Here's how the part is built. I have some questions about the finished solid (model axes, mm). Round coordinates to 2 decimals unless told otherwise and drop trailing zeros. Order: outer loops, then holes, each group sorted by start corner. A loop starts at its lowest first (then second) coordinate and runs counter-clockwise, first axis right, second up. Notation, with made-up numbers: (-23, -2) -> (6, -2) arc R18 cw to (6, 16) -> close; hole circle Ø1 at (-16, 71.25). An arc over 180 degrees is marked (long way). Use a Markdown table: item, result. Add a question column.
from build123d import *

# Parameters (mm, degrees)
SKETCH1_W           = 83
SKETCH1_H           = 327.5
BOSS_EXTRUDE1_DEPTH = 2
SKETCH2_R           = 1.6
CUT_EXTRUDE1_DEPTH  = 2
SKETCH3_R           = 1.93
CUT_EXTRUDE2_DEPTH  = 2
SKETCH4_W           = 116.407651787
SKETCH4_H           = 181.18090695
CUT_EXTRUDE3_DEPTH  = 10


with BuildPart() as part:
    # Sketch1 → Boss-Extrude1 (new body)
    with BuildSketch(Plane.XY):
        with Locations((41.5, 163.75)):
            Rectangle(SKETCH1_W, SKETCH1_H)
    extrude(amount=BOSS_EXTRUDE1_DEPTH)

    # Sketch2 → Cut-Extrude1 (cut)
    with BuildSketch(Plane.XY.offset(2)):
        with Locations((3.2, 314.9)):
            Circle(SKETCH2_R)
        with Locations((3.2, 308.5)):
            Circle(SKETCH2_R)
        with Locations((79.8, 314.9)):
            Circle(SKETCH2_R)
        with Locations((79.8, 308.5)):
            Circle(SKETCH2_R)
        with Locations((3.2, 240.925)):
            Circle(SKETCH2_R)
        with Locations((3.2, 234.525)):
            Circle(SKETCH2_R)
        with Locations((79.8, 240.925)):
            Circle(SKETCH2_R)
        with Locations((79.8, 234.525)):
            Circle(SKETCH2_R)
        with Locations((3.2, 166.95)):
            Circle(SKETCH2_R)
        with Locations((3.2, 160.55)):
            Circle(SKETCH2_R)
        with Locations((79.8, 166.95)):
            Circle(SKETCH2_R)
        with Locations((79.8, 160.55)):
            Circle(SKETCH2_R)
        with Locations((3.2, 92.975)):
            Circle(SKETCH2_R)
        with Locations((3.2, 86.575)):
            Circle(SKETCH2_R)
        with Locations((79.8, 92.975)):
            Circle(SKETCH2_R)
        with Locations((79.8, 86.575)):
            Circle(SKETCH2_R)
        with Locations((3.2, 19)):
            Circle(SKETCH2_R)
        with Locations((3.2, 12.6)):
            Circle(SKETCH2_R)
        with Locations((79.8, 19)):
            Circle(SKETCH2_R)
        with Locations((79.8, 12.6)):
            Circle(SKETCH2_R)
    extrude(amount=-CUT_EXTRUDE1_DEPTH, mode=Mode.SUBTRACT)

    # Sketch3 → Cut-Extrude2 (cut)
    with BuildSketch(Plane.XY.offset(2)):
        with Locations((41.5, 322.524)):
            Circle(SKETCH3_R)
        with Locations((41.5, 4.976)):
            Circle(SKETCH3_R)
    extrude(amount=-CUT_EXTRUDE2_DEPTH, mode=Mode.SUBTRACT)

    # Sketch4 → Cut-Extrude3 (cut)
    with BuildSketch(Plane.XY.offset(2)):
        with Locations((24.796174107, 254.340453475)):
            Rectangle(SKETCH4_W, SKETCH4_H)
    extrude(amount=-CUT_EXTRUDE3_DEPTH, mode=Mode.SUBTRACT)


solid = part.part
(1) If we mould it in two halves opening along Y, with no side actions, what happens to faces 1 (the flat face through (41, 83, 2)), 2 (the cylindrical face through (2.85, 11.04, 1.01))? For each: pulls with the +Y half, pulls with the -Y half, needs draft (parallel to the pull), parting line crosses it, or undercut.
(2) I want a section at B-B on y = 12.6. List the corners of the cut face in (x, z) for me.
(3) Please list where these lines run through material, in increasing order: probe 1 along Y at (x, z) = (3.2, 1.1) (3 decimals); probe 2 along X at (y, z) = (160.55, 1.35); probe 3 along Y at (x, z) = (78.5, 0.55). Write a range as from..to.
(4) I want a section at A-A on x = 79.8. List the corners of the cut face in (y, z) for me (3 decimals), and give its area (4 significant figures).
(5) I'm going to push a flat-ended pin straight in: P1, Ø2.5, axis at x = 3.2, y = 86.575, coming from the -Z side. Where does the tip first touch, or does it pass through?
Output:
| question | item | result |
|---|---|---|
| 1 | face 1 | needs draft |
| 1 | face 2 | undercut |
| 2 | outline | (0, 0) -> (1.6, 0) -> (1.6, 2) -> (0, 2) -> close; (4.8, 0) -> (78.2, 0) -> (78.2, 2) -> (4.8, 2) -> close; (81.4, 0) -> (83, 0) -> (83, 2) -> (81.4, 2) -> close |
| 3 | probe 1 | 0..11, 14.2..17.4, 20.6..84.975, 88.175..91.375, 94.575..158.95, 162.15..163.75 |
| 3 | probe 2 | 0..1.6, 4.8..78.2, 81.4..83 |
| 3 | probe 3 | 0..11.67, 13.53..18.07, 19.93..85.64, 87.51..92.04, 93.91..159.62, 161.48..163.75 |
| 4 | outline | (0, 0) -> (11, 0) -> (11, 2) -> (0, 2) -> close; (14.2, 0) -> (17.4, 0) -> (17.4, 2) -> (14.2, 2) -> close; (20.6, 0) -> (84.975, 0) -> (84.975, 2) -> (20.6, 2) -> close; (88.175, 0) -> (91.375, 0) -> (91.375, 2) -> (88.175, 2) -> close; (94.575, 0) -> (158.95, 0) -> (158.95, 2) -> (94.575, 2) -> close; (162.15, 0) -> (163.75, 0) -> (163.75, 2) -> (162.15, 2) -> close |
| 4 | area | 295.5 mm² |
| 5 | P1 | through |
